Work out the finished part from the listing and answer in its coordinate system (mm). A direction names the side the tool comes from. Give positions to 0.01 mm unless a question says otherwise; leave off trailing zeros. Order: outer loops, then holes, each group sorted by start corner. A loop starts at its lowest first (then second) coordinate and runs counter-clockwise, first axis right, second up.
```python
from build123d import *

# Parameters (mm, degrees)
F0_W     = 47.4850616275
F0_H     = 19.05
F0_W_2   = 16.0149383725
F0_W_3   = 19.05
F1_DEPTH = 63.5
F2_DEPTH = 25.4
F3_DEPTH = 7.9375


with BuildPart() as f1:
    # F0 (on Front) → F1 (new body, symmetric)
    with BuildSketch(Plane.XZ):
        with Locations((-17.5324691862, 0)):
            Rectangle(F0_W, F0_H)
        with Locations((33.2675308138, 0)):
            Rectangle(F0_W_2, F0_H)
        with Locations((15.7350616275, 0)):
            Rectangle(F0_W_3, F0_H)
    extrude(amount=F1_DEPTH, both=True)

    # F0 (on Front) → F2 (join, symmetric)
    with BuildSketch(Plane.XZ):
        with BuildLine():
            Line((6.2100616275, 9.525), (25.2600616275, 9.525))
            Line((25.2600616275, 9.525), (25.2600616275, 27.0002))
            ThreePointArc((25.2600616275, 27.0002), (29.9097414762, 38.2255201513), (41.1350616275, 42.8752))
            Line((41.1350616275, 42.8752), (60.325, 42.8752))
            Line((60.325, 42.8752), (60.325, 61.9252))
            Line((60.325, 61.9252), (41.1350616275, 61.9252))
            ThreePointArc((41.1350616275, 61.9252), (16.4393572946, 51.6959043329), (6.2100616275, 27.0002))
            Line((6.2100616275, 27.0002), (6.2100616275, 9.525))
        make_face()
        with Locations((15.7350616275, 0)):
            Rectangle(F0_W_3, F0_H)
        with Locations((33.2675308138, 0)):
            Rectangle(F0_W_2, F0_H)
        Polygon((60.325, 61.9252), (60.325, 42.8752), (60.325, 38.1), (98.117655005, 38.1), (98.2993766665, 66.675), (60.325, 66.675), align=None)
        Polygon((98.2993766665, 66.675), (98.117655005, 38.1), (111.125, 38.1), (111.125, 66.675), align=None)
    extrude(amount=F2_DEPTH, both=True)

    # F0 (on Front) → F3 (join, symmetric)
    with BuildSketch(Plane.XZ):
        with BuildLine():
            Line((-41.275, 9.525), (6.2100616275, 9.525))
            Line((6.2100616275, 9.525), (6.2100616275, 27.0002))
            ThreePointArc((6.2100616275, 27.0002), (16.4393572946, 51.6959043329), (41.1350616275, 61.9252))
            add(Edge.make_bspline(
                [(-41.275, 9.525), (-41.299830026, 60.5354448615), (25.0295793076, 63.5215594349), (41.1350616275, 61.9252)],
                knots=[0, 0, 0, 0, 97.6585849656, 97.6585849656, 97.6585849656, 97.6585849656], degree=3))
        make_face()
    extrude(amount=F3_DEPTH, both=True)


solid = f1.part
```
1. The part is cut by section B-B (x = 99.5). Write down the section's boundary in (y, z) (3 decimals), then the cut area to 3 significant figures.
Findings below:
outline: (-25.4, 38.1) - (25.4, 38.1) - (25.4, 66.675) - (-25.4, 66.675) - close
area: 1,450 mm2
2. The part is cut by section C-C (z = 0.5). Write down the section's boundary in (x, y) (3 decimals), then the cut area to 3 significant figures.
Findings below:
outline: (-41.275, -63.5) - (41.275, -63.5) - (41.275, 63.5) - (-41.275, 63.5) - close
area: 10,500 mm2
3. Which of the six approach directions +Z, -Z, +X, -X, +Y, -Y give full straight-line access (tool end or side, diameter ignored) to faces 1 (the face through (85, 0, 38.1)), 2 (the face through (-10, 7.938, 31)), 3 (the face through (6.21, -17, 18))?
Findings below:
face 1: -Z, +X, +Y, -Y
face 2: +Z, -X, +Y
face 3: +Z, -X, -Y
4. The part is cut by section A-A (y = -16.5). Write down the section's boundary in (x, z) (3 decimals).
Findings below:
outline: (-41.275, -9.525) - (41.275, -9.525) - (41.275, 9.525) - (25.26, 9.525) - (25.26, 27) arc R15.875 cw to (41.135, 42.875) - (60.325, 42.875) - (60.325, 38.1) - (111.125, 38.1) - (111.125, 66.675) - (60.325, 66.675) - (60.325, 61.925) - (41.135, 61.925) arc R34.925 ccw to (6.21, 27) - (6.21, 9.525) - (-41.275, 9.525) - close
5. Given P1, Ø5.5, axis at y = -17, z = -3, coming from the +X side (3 decimals); P2, Ø2, axis at x = 6.5, z = 20, coming from the -Y side; P3, Ø12, axis at x = 29.5, y = 12.5, coming from the +Z side, each flat-ended and moving along its own axis, determine where each tip first touches the part or whether it passes through.
Findings below:
P1: stops at x = 41.275
P2: stops at y = -25.4
P3: stops at z = 62.23
6. Straight lines are drawn through the part: probe 1 along Y at (x, z) = (79.5, 56); probe 2 along Z at (x, y) = (11, 58.5) (3 decimals); probe 3 along Z at (x, y) = (90, 18) (3 decimals). For each, find the intervals that lie inside material, in ascending order.
Findings below:
probe 1: y = -25.4 to 25.4
probe 2: z = -9.525 to 9.525
probe 3: z = 38.1 to 66.675
